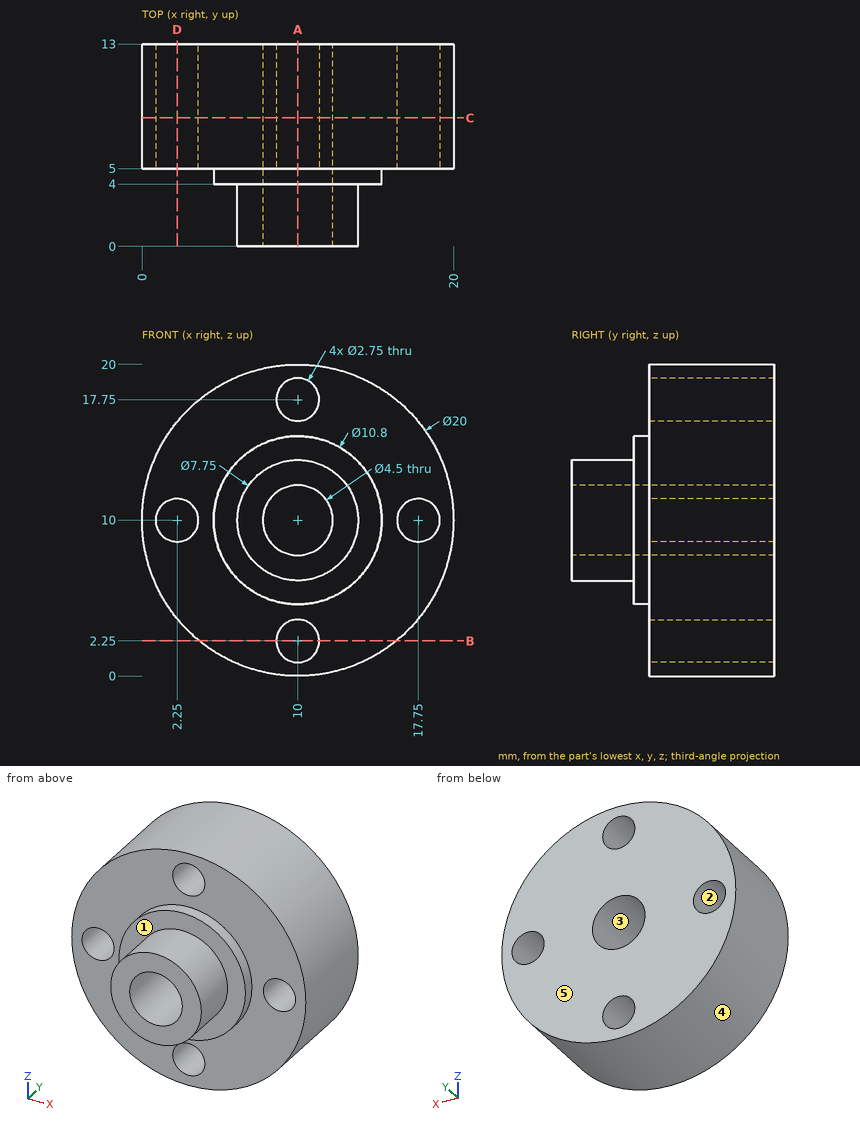
Job drawing, mm, ordinate dimensions from the low corner. One solid piece. A direction names the side the tool comes from. Coordinates: 2 decimals unless noted, no trailing zeros. Order: outer loops, then holes, each group sorted by start corner. A loop starts at its lowest first (then second) coordinate and runs counter-clockwise, first axis right, second up. Notation, with made-up numbers: (-5, 62.25) - (13, 62.25) arc R32 cw to (13, 95.25) - close; hole circle Ø8 at (-33.75, 3.5). An arc over 180 degrees is marked (long way). Write each question's results on one line, items separated by ' | '. Start each with the question number.
Item 1: Band-saw the part on D-D on x = 2.25. Write the cut outline in (y, z) (3 decimals), and give its area (3 significant figures).
Item 2: Tool access for the marked faces 1 and 2: list every direction of +Z, -Z, +X, -X, +Y, -Y with a clear straight run to the whole face (end or side of a thin tool).
Item 3: Flat gauge pins, fed straight in: pin 1 (1 mm diameter, centred on y = 10.5, z = 8.5, fed in from +X); pin 2 (2.5 mm diameter, centred on x = 2.25, z = 10, fed in from -Y); pin 3 (4.5 mm diameter, centred on x = 17.75, z = 10, fed in from -Y); pin 4 (3 mm diameter, centred on x = 14, y = 11.5, fed in from +Z). Where does each tip first touch, or does it go through?
Item 4: Band-saw the part on B-B on z = 2.25. Write the cut outline in (x, y) (3 decimals), and give its area (3 significant figures).
Item 5: Mould opens along Z. For the marked faces 3, 4 and 5 say: released by +Z, released by -Z, zero draft, split by the parting line, or undercut.
Item 6: Band-saw the part on A-A on x = 10. Write the cut outline in (y, z) (3 decimals).
Item 7: Wall check: probe 1 along Z at (x, y) = (10, 4.5); probe 2 along Z at (x, y) = (10, 3.5) (3 decimals); probe 3 along Y at (x, z) = (15.5, 13). Give the ranges that are in metal, low to high. Write a range as [from, to].
Item 8: Band-saw the part on C-C on y = 8.25. Write the cut outline in (x, z) (3 decimals).
Numbers:
1) outline: (5, 3.68) - (13, 3.68) - (13, 8.625) - (5, 8.625) - close; (5, 11.375) - (13, 11.375) - (13, 16.32) - (5, 16.32) - close | area: 79.1 mm^2
2) face 1: -Y | face 2: +Y, -Y
3) pin 1: x = 19.95 | pin 2: through | pin 3: y = 5 | pin 4: z = 19.68
4) outline: (3.68, 5) - (8.625, 5) - (8.625, 13) - (3.68, 13) - close; (11.375, 5) - (16.32, 5) - (16.32, 13) - (11.375, 13) - close | area: 79.1 mm^2
5) face 3: undercut | face 4: split by the parting line | face 5: zero draft
6) outline: (0, 6.125) - (4, 6.125) - (4, 4.6) - (5, 4.6) - (5, 3.625) - (13, 3.625) - (13, 7.75) - (0, 7.75) - close; (0, 12.25) - (13, 12.25) - (13, 16.375) - (5, 16.375) - (5, 15.4) - (4, 15.4) - (4, 13.875) - (0, 13.875) - close; (5, 0) - (13, 0) - (13, 0.875) - (5, 0.875) - close; (5, 19.125) - (13, 19.125) - (13, 20) - (5, 20) - close
7) probe 1: [4.6, 7.75], [12.25, 15.4] | probe 2: [6.125, 7.75], [12.25, 13.875] | probe 3: [5, 13]
8) outline: circle Ø20 at (10, 10); hole circle Ø2.75 at (2.25, 10); hole circle Ø4.5 at (10, 10); hole circle Ø2.75 at (10, 2.25); hole circle Ø2.75 at (10, 17.75); hole circle Ø2.75 at (17.75, 10)
